Geometry: final body of the model. Coordinates: model frame, mm. A direction names the side the tool comes from. Coordinates: 2 decimals unless noted, no trailing zeros. Loops run counter-clockwise (first coordinate to the right, second up) from the corner with the lowest first, then second, coordinate; pieces in that order, holes last. Notation, with made-up numbers: (33, -28) - (58, -28) arc R28 cw to (58, -4) - close; hole circle Ø5 at (70, 22.5). An arc over 180 degrees is marked (long way). Answer in a Markdown table with one row per item.
from build123d import *

# Parameters (mm, degrees)
BOSS_EXTRUDE1_DEPTH = 3.175
SKETCH2_R           = 4
CUT_EXTRUDE3_DEPTH  = 4.175
SKETCH3_R           = 1.5
CUT_EXTRUDE4_DEPTH  = 4.175


with BuildPart() as part:
    # Sketch1 → Boss-Extrude1 (new body)
    with BuildSketch(Plane(origin=(0, 0, 0), x_dir=(1, 0, 0), z_dir=(0, 1, 0))):
        with BuildLine():
            Line((96.897642196, 30.55170923), (95.120945792, 27.138707192))
            ThreePointArc((95.120945792, 27.138707192), (77.57215373, 15.134042144), (57.841053042, 23.055894918))
            Line((57.841053042, 23.055894918), (17.668897816, 70.931205231))
            ThreePointArc((17.668897816, 70.931205231), (13.19211244, 74.548556577), (7.682670578, 76.213755798))
            ThreePointArc((7.682670578, 76.213755798), (-76.6, 0), (7.682670578, -76.213755798))
            ThreePointArc((7.682670578, -76.213755798), (13.19211244, -74.548556577), (17.668897816, -70.931205231))
            Line((17.668897816, -70.931205231), (57.841053042, -23.055894918))
            ThreePointArc((57.841053042, -23.055894918), (77.57215373, -15.134042144), (95.120945792, -27.138707192))
            Line((95.120945792, -27.138707192), (96.897642196, -30.55170923))
            ThreePointArc((96.897642196, -30.55170923), (101.6, 0), (96.897642196, 30.55170923))
        make_face()
        with BuildLine():
            Line((5.98413489, 53.742086889), (26.146554137, 29.713451316))
            ThreePointArc((26.146554137, 29.713451316), (27.003715662, 15.442284424), (13.595828747, 10.479472842))
            Line((13.595828747, 10.479472842), (-31.001636142, 23.479472842))
            ThreePointArc((-31.001636142, 23.479472842), (-39.421951774, 32.705058554), (-35.081142025, 44.417040359))
            ThreePointArc((-35.081142025, 44.417040359), (-18.647504357, 53.439971756), (-0.16796068, 56.599750788))
            ThreePointArc((-0.16796068, 56.599750788), (3.225963821, 55.855256817), (5.98413489, 53.742086889))
        make_face(mode=Mode.SUBTRACT)
        with BuildLine():
            Line((5.98413489, -53.742086889), (26.146554137, -29.713451316))
            ThreePointArc((26.146554137, -29.713451316), (27.003715662, -15.442284424), (13.595828747, -10.479472842))
            Line((13.595828747, -10.479472842), (-31.001636142, -23.479472842))
            ThreePointArc((-31.001636142, -23.479472842), (-39.421951774, -32.705058554), (-35.081142025, -44.417040359))
            ThreePointArc((-35.081142025, -44.417040359), (-18.647504357, -53.439971756), (-0.16796068, -56.599750788))
            ThreePointArc((-0.16796068, -56.599750788), (3.225963821, -55.855256817), (5.98413489, -53.742086889))
        make_face(mode=Mode.SUBTRACT)
    extrude(amount=BOSS_EXTRUDE1_DEPTH)

    # Sketch2 → Cut-Extrude3 (cut, through all)
    with BuildSketch(Plane(origin=(0, 0, 0), x_dir=(1, 0, 0), z_dir=(0, 1, 0))):
        with Locations((0.378636362, 0)):
            Circle(SKETCH2_R)
    extrude(amount=CUT_EXTRUDE3_DEPTH, mode=Mode.SUBTRACT)

    # Sketch3 → Cut-Extrude4 (cut, through all)
    with BuildSketch(Plane(origin=(0, 0, 0), x_dir=(1, 0, 0), z_dir=(0, 1, 0))):
        with Locations((-12.321363638, 0)):
            Circle(SKETCH3_R)
        with Locations((13.078636362, 0)):
            Circle(SKETCH3_R)
    extrude(amount=CUT_EXTRUDE4_DEPTH, mode=Mode.SUBTRACT)


solid = part.part
(1) Pull-direction query (X, two-part tool) for faces 3 (the face through (15.92, 1.57, 41.9)), 4 (the face through (101.6, 1.6, 0.4)), 5 (the face through (-9, 3.175, -1)); classes: pulls with the +X half, pulls with the -X half, needs draft (parallel to the pull), parting line crosses it, or undercut.
Verdict:
| item | result |
|---|---|
| face 3 | undercut |
| face 4 | pulls with the +X half |
| face 5 | needs draft |
(2) Access query for faces 1 (the face through (-39.385, 1.565, 32.525)), 2 (the face through (13.264, 1.565, -74.51)). Directions: +Z, -Z, +X, -X, +Y, -Y. A direction counts if a zero-diameter tool reaches every point of the face in a straight line with its end or side. Return the directions, or none.
Verdict:
| item | result |
|---|---|
| face 1 | +Y, -Y |
| face 2 | -Z, +X, +Y, -Y |
(3) Cut plane C-C on z = 42. Output: boundary loops of the cut face in (x, y) (3 decimals), then the cut area to 3 significant figures.
Verdict:
| item | result |
|---|---|
| outline | (-64.059, 0) - (-37.39, 0) - (-37.39, 3.175) - (-64.059, 3.175) - close; (15.837, 0) - (41.945, 0) - (41.945, 3.175) - (15.837, 3.175) - close |
| area | 168 mm² |
(4) First-contact query: pin 1 Ø1 at (y, z) = (1.5, 34.5) entering from +X; pin 2 Ø1.5 at (x, y) = (77, 2) entering from -Z. Flat tips, straight axial feed; report the tip coordinate or a pass-through.
Verdict:
| item | result |
|---|---|
| pin 1 | stops at x = 48.66 |
| pin 2 | stops at z = -15.15 |
(5) Cut plane D-D on x = 38. Output: boundary loops of the cut face in (y, z) (3 decimals), then the cut area to 3 significant figures.
Verdict:
| item | result |
|---|---|
| outline | (0, -46.702) - (3.175, -46.702) - (3.175, 46.702) - (0, 46.702) - close |
| area | 297 mm² |
(6) Ray query, probe 1 along X at (y, z) = (0.35, 0); probe 2 along Z at (x, y) = (-24, 2.75); probe 3 along Z at (x, y) = (-15.5, 1.85). Return the intervals inside material, ascending.
Verdict:
| item | result |
|---|---|
| probe 1 | x = -76.6 to -13.82, -10.82 to -3.62, 4.38 to 11.58, 14.58 to 101.6 |
| probe 2 | z = -72.74 to -51.26, -21.44 to 21.44, 51.26 to 72.74 |
| probe 3 | z = -75.02 to -54.44, -18.96 to 18.96, 54.44 to 75.02 |
(7) Cut plane A-A on y = 1.7. Output: boundary loops of the cut face in (x, z).
Verdict:
| item | result |
|---|---|
| outline | (7.68, -76.21) arc R15 ccw to (17.67, -70.93) - (57.84, -23.06) arc R22.55 cw to (95.12, -27.14) - (96.9, -30.55) arc R101.6 ccw to (96.9, 30.55) - (95.12, 27.14) arc R22.55 cw to (57.84, 23.06) - (17.67, 70.93) arc R15 ccw to (7.68, 76.21) arc R76.6 ccw (long way) to start; hole (-35.08, -44.42) arc R56.6 ccw to (-0.17, -56.6) arc R8 ccw to (5.98, -53.74) - (26.15, -29.71) arc R12 ccw to (13.6, -10.48) - (-31, -23.48) arc R12 ccw to start; hole (-35.08, 44.42) arc R12 ccw to (-31, 23.48) - (13.6, 10.48) arc R12 ccw to (26.15, 29.71) - (5.98, 53.74) arc R8 ccw to (-0.17, 56.6) arc R56.6 ccw to start; hole circle Ø3 at (-12.32, 0); hole circle Ø8 at (0.38, 0); hole circle Ø3 at (13.08, 0) |
(8) Cut plane B-B on z = -50. Output: boundary loops of the cut face in (x, y) (3 decimals).
Verdict:
| item | result |
|---|---|
| outline | (-58.031, 0) - (-26.525, 0) - (-26.525, 3.175) - (-58.031, 3.175) - close; (9.124, 0) - (35.232, 0) - (35.232, 3.175) - (9.124, 3.175) - close |
